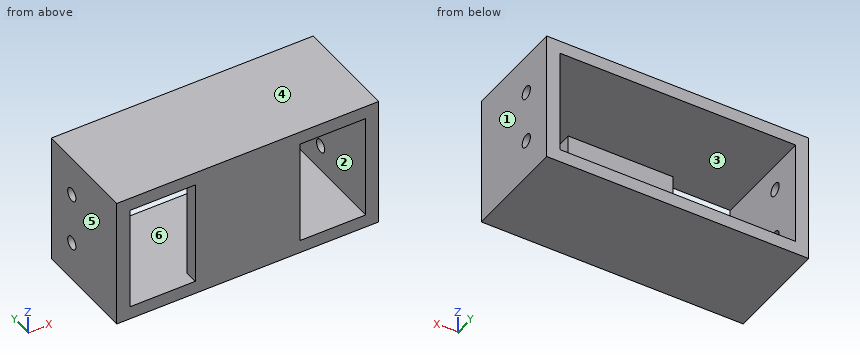
from build123d import *

# Parameters (mm, degrees)
SKETCH1_W           = 100
SKETCH1_H           = 50
SKETCH1_W_2         = 90
SKETCH1_H_2         = 40
BOSS_EXTRUDE1_DEPTH = 40
SKETCH3_W           = 40
SKETCH3_H           = 40
BOSS_EXTRUDE2_DEPTH = 5
SKETCH4_R           = 2.5
CUT_EXTRUDE1_DEPTH  = 116


with BuildPart() as part:
    # Sketch1 → Boss-Extrude1 (new body)
    with BuildSketch(Plane(origin=(0, 0, 0), x_dir=(1, 0, 0), z_dir=(0, 1, 0))):
        with Locations((11.771561772, 25)):
            Rectangle(SKETCH1_W, SKETCH1_H)
        with Locations((11.771561772, 25)):
            Rectangle(SKETCH1_W_2, SKETCH1_H_2, mode=Mode.SUBTRACT)
    extrude(amount=BOSS_EXTRUDE1_DEPTH)

    # Sketch3 → Boss-Extrude2 (add)
    with BuildSketch(Plane(origin=(0, 0, 0), x_dir=(-1, 0, 0), z_dir=(0, -1, 0))):
        with Locations((-11.771561772, 25)):
            Rectangle(SKETCH3_W, SKETCH3_H)
    extrude(amount=-BOSS_EXTRUDE2_DEPTH)

    # Sketch4 → Cut-Extrude1 (cut)
    with BuildSketch(Plane.ZY.offset(38.228438228)):
        with Locations((-35, 27.5)):
            Circle(SKETCH4_R)
        with Locations((-15, 27.5)):
            Circle(SKETCH4_R)
    extrude(amount=-CUT_EXTRUDE1_DEPTH, mode=Mode.SUBTRACT)


solid = part.part
Design review of the part built by this model. Coordinates are the model's own, in mm. Face numbers are marked on the shaded views. A direction names the side the tool comes from. Give positions to 0.01 mm unless a question says otherwise; leave off trailing zeros. Order: outer loops, then holes, each group sorted by start corner. A loop starts at its lowest first (then second) coordinate and runs counter-clockwise, first axis right, second up.
1. Mouldability with a two-part tool opening along X and no side actions: class the marked faces 4, 5 and 6 as +X half, -X half, draft (parallel to the pull), parting line (faces both ways), or undercut.
Solution:
face 4: draft
face 5: -X half
face 6: undercut
2. Add section A-A, the plane z = -24. State the section outline as (x, y) points, then the cut area to 3 significant figures.
Solution:
outline: (-38.23, 0) - (-33.23, 0) - (-33.23, 40) - (-38.23, 40) - close; (-8.23, 0) - (31.77, 0) - (31.77, 5) - (-8.23, 5) - close; (56.77, 0) - (61.77, 0) - (61.77, 40) - (56.77, 40) - close
area: 600 mm2
3. Add section B-B, the plane y = 27.5. State the section outline as (x, z) points, then the cut area to 3 significant figures.
Solution:
outline: (-38.23, -50) - (61.77, -50) - (61.77, -37.5) - (56.77, -37.5) - (56.77, -45) - (-33.23, -45) - (-33.23, -37.5) - (-38.23, -37.5) - close; (-38.23, -32.5) - (-33.23, -32.5) - (-33.23, -17.5) - (-38.23, -17.5) - close; (-38.23, -12.5) - (-33.23, -12.5) - (-33.23, -5) - (56.77, -5) - (56.77, -12.5) - (61.77, -12.5) - (61.77, 0) - (-38.23, 0) - close; (56.77, -32.5) - (61.77, -32.5) - (61.77, -17.5) - (56.77, -17.5) - close
area: 1,300 mm2
4. For pin 1 Ø8 at (x, z) = (29, -31.5) entering from +Y, flat-tipped, find the tip position at first contact; note if it passes through.
Solution:
pin 1: stops at y = 5
5. To check wall thickness, follow L1, parallel to X at y = 4, z = -11; L2, parallel to Y at x = 60, z = -35; L3, parallel to X at y = 5.5, z = -13. State the ranges of each line that lie inside material, in increasing order.
Solution:
L1: x = -38.23 to -33.23, -8.23 to 31.77, 56.77 to 61.77
L2: y = 0 to 25, 30 to 40
L3: x = -38.23 to -33.23, 56.77 to 61.77
6. Add section D-D, the plane x = 46. State the section outline as (y, z) points.
Solution:
outline: (0, -50) - (40, -50) - (40, -45) - (0, -45) - close; (0, -5) - (40, -5) - (40, 0) - (0, 0) - close
7. Tool access review of the marked faces 1, 2 and 3: name each direction out of +Z, -Z, +X, -X, +Y, -Y from which nothing blocks a thin tool from reaching the whole face with its end or side.
Solution:
face 1: +Z, -Z, +X, +Y, -Y
face 2: +Y, -Y
face 3: +Y
8. Add section C-C, the plane z = -15. State the section outline as (x, y) points, then the cut area to 3 significant figures.
Solution:
outline: (-38.23, 0) - (-33.23, 0) - (-33.23, 25) - (-38.23, 25) - close; (-38.23, 30) - (-33.23, 30) - (-33.23, 40) - (-38.23, 40) - close; (-8.23, 0) - (31.77, 0) - (31.77, 5) - (-8.23, 5) - close; (56.77, 0) - (61.77, 0) - (61.77, 25) - (56.77, 25) - close; (56.77, 30) - (61.77, 30) - (61.77, 40) - (56.77, 40) - close
area: 550 mm2
